Study the drawing (mm; zero at the part's minimum x, y, z) and answer. A direction names the side the tool comes from. Coordinates: 2 decimals unless noted, no trailing zeros. Order: outer loops, then holes, each group sorted by start corner. A loop starts at its lowest first (then second) coordinate and runs counter-clockwise, first axis right, second up. Notation, with made-up numbers: (-21.75, 80.25) -> (2.25, 80.25) arc R20 ccw to (2.25, 119.25) -> close; hole circle Ø11 at (-2, 10.25). An arc over 180 degrees is marked (long way). Answer as CSV lines item,"result". Start each with the question number.
Item 1: Straight lines are drawn through the part: L1, parallel to X at y = 8, z = 16.25 (1 decimal); L2, parallel to Y at x = 6, z = 7; L3, parallel to Y at x = 78.5, z = 2. For each, find the intervals that lie inside material, in ascending order.
Item 2: Section D-D (y = 22) is taken. Write down the section's boundary in (x, z) (1 decimal).
Item 3: For a pull along X with two mould halves and no side action, classify the marked faces 1, 2, 3 and 4 as pulls with the +X half, pulls with the -X half, needs draft (parallel to the pull), parting line crosses it, or undercut.
Item 4: Each of these flat-tipped pins is pushed along its axis until it touches: pin 1 Ø10 at (y, z) = (28, 14) entering from -X; pin 2 Ø7.5 at (x, z) = (60, 15) entering from -Y; pin 3 Ø8.5 at (x, z) = (7.5, 8.5) entering from +Y. Where does it stop, or does it pass through?
Item 5: Section C-C (x = 74.5) is taken. Write down the section's boundary in (y, z), then the cut area to 3 significant figures.
Item 6: Which of the six approach directions +Z, -Z, +X, -X, +Y, -Y give full straight-line access (tool end or side, diameter ignored) to the marked faces 5, 6, 7, 8 and 9?
Item 7: Section A-A (y = 10.5) is taken. Write down the section's boundary in (x, z) (1 decimal), then the cut area to 3 significant figures.
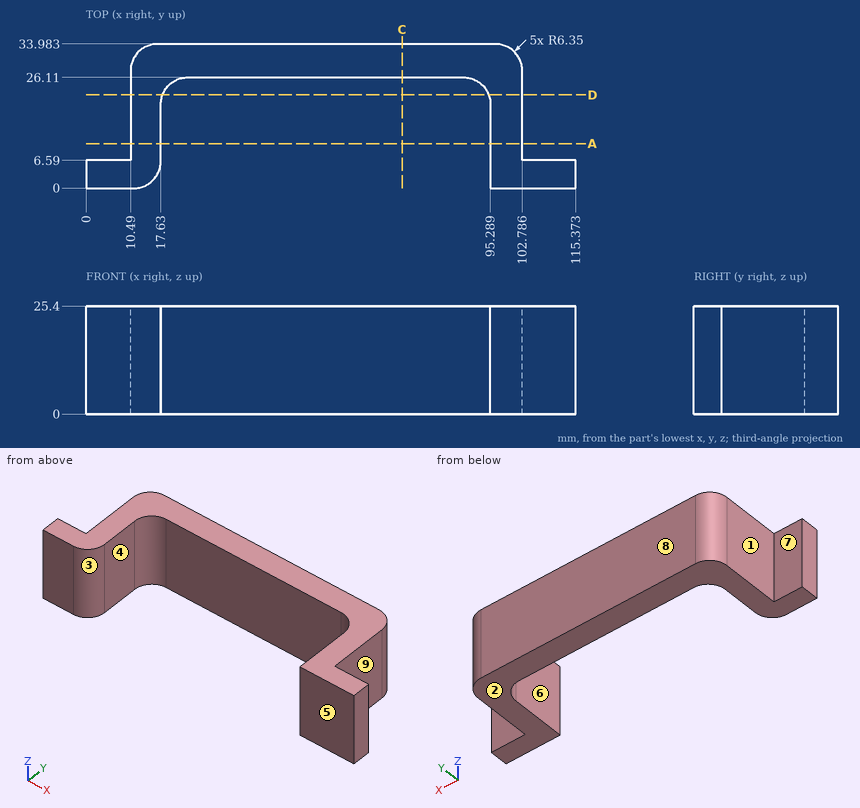
Checked values:
1,L1,"x = 10.5 to 17.6, 95.3 to 102.8"
1,L2,"y = 0 to 6.59"
1,L3,"y = 26.11 to 33.98"
2,outline,"(10.5, 0) -> (18, 0) -> (18, 25.4) -> (10.5, 25.4) -> close; (94.9, 0) -> (102.8, 0) -> (102.8, 25.4) -> (94.9, 25.4) -> close"
3,face 1,"pulls with the -X half"
3,face 2,"needs draft"
3,face 3,"undercut"
3,face 4,"undercut"
4,pin 1,"stops at x = 10.49"
4,pin 2,"stops at y = 26.11"
4,pin 3,"stops at y = 31.43"
5,outline,"(26.11, 0) -> (33.98, 0) -> (33.98, 25.4) -> (26.11, 25.4) -> close"
5,area,"200 mm^2"
6,face 5,"+Z, -Z, +X, -X, -Y"
6,face 6,"+Z, -Z, -Y"
6,face 7,"+Z, -Z, -X, +Y"
6,face 8,"+Z, -Z, +X, -X, +Y"
6,face 9,"+Z, -Z, +X, +Y"
7,outline,"(10.5, 0) -> (17.6, 0) -> (17.6, 25.4) -> (10.5, 25.4) -> close; (95.3, 0) -> (102.8, 0) -> (102.8, 25.4) -> (95.3, 25.4) -> close"
7,area,"372 mm^2"
